Check sheet for the modelled part. Datum: model origin and axes. Units: mm. Coordinates: 2 decimals unless noted, no trailing zeros. Loops run counter-clockwise (first coordinate to the right, second up) from the corner with the lowest first, then second, coordinate; pieces in that order, holes last. Notation, with made-up numbers: M 40,61.5 L 62,61.5 A18 ccw 62,69.5 Z; hole C 9.25,-9 d10. An arc over 180 degrees is marked long. Answer in a Markdown table with one row per item. Add a question column.
```python
from build123d import *

# Parameters (mm, degrees)
BOSS_EXTRUDE1_DEPTH   = 5.08
SKETCH2_R             = 19.05
SKETCH2_R_2           = 5.55625
CUT_EXTRUDE1_DEPTH    = 6.08
F_6_CLEARANCE_HOLE1_D = 3.7973
SKETCH5_R             = 19.05
SKETCH5_R_2           = 8.73125
SKETCH5_R_3           = 5.55625
BOSS_EXTRUDE2_DEPTH   = 5.08


with BuildPart() as part:
    # Sketch1 → Boss-Extrude1 (new body)
    with BuildSketch(Plane.XY):
        Polygon((-36.785608025, 9.921141176), (36.785608025, 9.921141176), (75.212399069, -132.557717648), (38.426791044, -142.478858824), (-38.426791044, -142.478858824), (-75.212399069, -132.557717648), align=None)
    extrude(amount=BOSS_EXTRUDE1_DEPTH)

    # Sketch2 → Cut-Extrude1 (cut, through all)
    with BuildSketch(Plane.XY.offset(5.08)):
        with Locations((0, -73.157410737)):
            Circle(SKETCH2_R)
        with Locations((-36.5125, -73.157410737)):
            Circle(SKETCH2_R_2)
        with Locations((36.5125, -73.157410737)):
            Circle(SKETCH2_R_2)
    extrude(amount=-CUT_EXTRUDE1_DEPTH, mode=Mode.SUBTRACT)

    # #6 Clearance Hole1 (through all)
    with Locations(Plane.XY.offset(5.08)):
        with Locations((50.205500939, -112.994549553), (-50.205500939, -112.994549553), (-23.749124469, -14.899594819), (23.749124469, -14.899594819)):
            Hole(F_6_CLEARANCE_HOLE1_D / 2)

    # Sketch5 → Boss-Extrude2 (add)
    with BuildSketch(Plane.XY.offset(5.08)):
        with Locations((0, -73.157410737)):
            Circle(SKETCH5_R)
        with Locations((0, -73.157410737)):
            Circle(SKETCH5_R_2, mode=Mode.SUBTRACT)
        with Locations((36.5125, -73.157410737)):
            Circle(SKETCH5_R_3)
        with Locations((-36.5125, -73.157410737)):
            Circle(SKETCH5_R_3)
    extrude(amount=-BOSS_EXTRUDE2_DEPTH)


solid = part.part
```
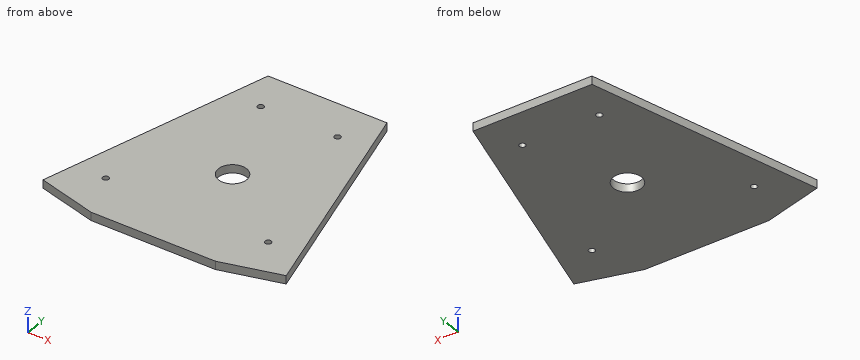
Q1. Cross-section at B-B (z = 1.2). Record the cut outline in (x, y), plus the area to 3 significant figures.
Q2. Cross-section at D-D (x = -43). Record the cut outline in (y, z), plus the area to 3 significant figures.
Q3. Cross-section at C-C (y = -52.5). Record the cut outline in (x, z), plus the area to 3 significant figures.
Q4. Go/stop test with flat-tipped pins: pin 1 (15.5 mm diameter, centred on x = 0, y = -73.16, fed in from +Z); pin 2 (2 mm diameter, centred on y = -41.5, z = 4.5, fed in from -X); pin 3 (2 mm diameter, centred on y = -37, z = 0.5, fed in from -X); pin 4 (2 mm diameter, centred on y = -87.5, z = 2.5, fed in from -X). Record where each tip stops, or that it passes through.
Q5. Cross-section at A-A (x = 0). Record the cut outline in (y, z).
Q6. Thickness scan on L1, parallel to X at y = -13.5, z = 3.45; L2, parallel to X at y = -16.5, z = 4.35; L3, parallel to X at y = -68.5, z = 3.6. Record the ranges inside material, lowest first.
Answer key:
| question | item | result |
|---|---|---|
| 1 | outline | M -75.21,-132.56 L -38.43,-142.48 L 38.43,-142.48 L 75.21,-132.56 L 36.79,9.92 L -36.79,9.92 Z; hole C -50.21,-112.99 d3.8; hole C -23.75,-14.9 d3.8; hole C 0,-73.16 d17.46; hole C 23.75,-14.9 d3.8; hole C 50.21,-112.99 d3.8 |
| 1 | area | 16,800 mm^2 |
| 2 | outline | M -141.25,0 L -13.12,0 L -13.12,5.08 L -141.25,5.08 Z |
| 2 | area | 651 mm^2 |
| 3 | outline | M -53.62,0 L 53.62,0 L 53.62,5.08 L -53.62,5.08 Z |
| 3 | area | 545 mm^2 |
| 4 | pin 1 | through |
| 4 | pin 2 | x = -50.92 |
| 4 | pin 3 | x = -49.71 |
| 4 | pin 4 | x = -63.33 |
| 5 | outline | M -142.48,0 L -81.89,0 L -81.89,5.08 L -142.48,5.08 Z; M -64.43,0 L 9.92,0 L 9.92,5.08 L -64.43,5.08 Z |
| 6 | L1 | -43.1 to -25.03, -22.47 to 22.47, 25.03 to 43.1 |
| 6 | L2 | -43.91 to -24.77, -22.73 to 22.73, 24.77 to 43.91 |
| 6 | L3 | -57.94 to -7.39, 7.39 to 57.94 |
